from build123d import *

# Parameters (mm, degrees)
F1_DEPTH = 3
F3_COUNT = 14
F4_R     = 2.5
F5_DEPTH = 3


with BuildPart() as f1:
    # F0 (on Front) → F1 (new body)
    with BuildSketch(Plane.XZ):
        with BuildLine():
            add(Edge.make_bspline(
                [(-1.125, 8.6773771959), (-0.7, 9.2234754838), (-0.6486890223, 9.6124048493), (-0.5, 10.4880884817), (0, 10.75)],
                knots=[0, 0, 0, 0, 0.4967173091, 1, 1, 1, 1], degree=3))
            ThreePointArc((-1.125, 8.6773771959), (0, -8.75), (1.125, 8.6773771959))
            add(Edge.make_bspline(
                [(1.125, 8.6773771959), (0.7, 9.2234754838), (0.6486890223, 9.6124048493), (0.5, 10.4880884817), (0, 10.75)],
                knots=[0, 0, 0, 0, 0.4967173091, 1, 1, 1, 1], degree=3))
        make_face()
    extrude(amount=F1_DEPTH)

    # F3: F1 ×14 about axis
    f3_axis = Axis((0, 2.5461101905, 0), (0, 1, 0))


with BuildPart() as f1_1:
    add(f1.part)
    for i in range(1, F3_COUNT):
        add(f1.part.rotate(f3_axis, i * 360 / F3_COUNT))

    # F4 (on face) → F5 (cut, through all)
    with BuildSketch(Plane.XZ.offset(3)):
        Circle(F4_R)
    extrude(amount=-F5_DEPTH, mode=Mode.SUBTRACT)


solid = f1_1.part
Geometry check sheet. Reference: the model listing, model coordinates, mm. A direction names the side the tool comes from. Round coordinates to 2 decimals unless told otherwise and drop trailing zeros. Loops run counter-clockwise (first coordinate to the right, second up) from the corner with the lowest first, then second, coordinate; pieces in that order, holes last.
Item 1: Cross-section at B-B on x = -1.5. Record the boundary of the cut face in (y, z).
Item 2: Mould release check, pull along Z, two halves, no side actions. Record for faces 5 (the cylindrical face through (-1.936, -1.479, 8.533)), 6 (the cylindrical face through (1.936, -1.479, -8.533)), 7 (the cylindrical face through (-0.54, -1.52, -2.44)): pulls with the +Z half, pulls with the -Z half, needs draft (parallel to the pull), parting line crosses it, or undercut.
Item 3: Access from +Z, -Z, +X, -X, +Y, -Y to the whole of each face (thin tool, end or side, straight path). Record for faces 1 (the cylindrical face through (-7.878, -1.479, 3.807)), 2 (the cylindrical face through (1.958, -1.479, 8.528)), 3 (the cylindrical face through (7.878, -1.479, -3.807)), 4 (the cylindrical face through (-1.958, -1.479, -8.528)).
Item 4: Cross-section at C-C on z = -9. Count the separate pieces of the cut face and the enclosed holes in it, then the cut area to 3 significant figures.
Item 5: Thickness scan on line 1 (Z direction, x = 8, y = -2.55); line 2 (X direction, y = -1.2, z = -0.75); line 3 (X direction, y = -0.2, z = -1.25). Record the ranges inside material, lowest first.
Item 6: Gauge pin test, flat end, axial feed: pin 1 (8 mm diameter, centred on x = -6, z = -8, fed in from -Y). Record the tip position at first contact, or that the pin passes through.
Item 7: Cross-section at A-A on z = 0. Record the boundary of the cut face in (x, y), then the cut area to 3 significant figures.
Item 8: Cross-section at D-D on z = -3.75. Record the boundary of the cut face in (x, y).
Answer sheet:
1. outline: (-3, -8.62) - (0, -8.62) - (0, -2) - (-3, -2) - close; (-3, 2) - (0, 2) - (0, 8.62) - (-3, 8.62) - close
2. face 5: pulls with the +Z half
2. face 6: pulls with the -Z half
2. face 7: undercut
3. face 1: -X, +Y, -Y
3. face 2: +Z, +Y, -Y
3. face 3: +X, +Y, -Y
3. face 4: -Z, +Y, -Y
4. separate pieces: 3
4. enclosed holes: 0
4. area: 12.9 mm2
5. line 1: z = -6.8 to -5.58, -3.54 to 3.54, 5.58 to 6.8
5. line 2: x = -8.72 to -2.38, 2.38 to 8.72
5. line 3: x = -9.1 to -2.17, 2.17 to 9.1
6. pin 1: stops at y = -3
7. outline: (-8.75, -3) - (-2.5, -3) - (-2.5, 0) - (-8.75, 0) - close; (2.5, -3) - (8.75, -3) - (8.75, 0) - (2.5, 0) - close
7. area: 37.5 mm2
8. outline: (-7.91, -3) - (7.91, -3) - (7.91, 0) - (-7.91, 0) - close
